Geometry check sheet. Reference: the model listing, model coordinates, mm. A direction names the side the tool comes from. Coordinates: 2 decimals unless noted, no trailing zeros. Loops run counter-clockwise (first coordinate to the right, second up) from the corner with the lowest first, then second, coordinate; pieces in that order, holes last. Notation, with made-up numbers: (14, 30) - (55, 30) arc R17 cw to (55, 47) - close; hole circle Ø3 at (58, 22). An arc over 180 degrees is marked (long way). Write each question's results on one line, items separated by ' | '. Start each with the question number.
(1) Sectioned sample at D-D (y = 32.5). Enter the section's corners in (x, z), plus the area to 3 significant figures.
(2) Material ranges on probe 1 along Y at (x, z) = (50, 9); probe 2 along X at (y, z) = (68, 27.5); probe 3 along Y at (x, z) = (24.5, 2.5), recorded low to high.
(3) Mould release check, pull along Y, two halves, no side actions. Record for faces 1 (the face through (55, 78, 16)), 2 (the face through (53, 45, 17)), 3 (the face through (23, 41, -4)), 4 (the face through (54, 11, 16)): pulls with the +Y half, pulls with the -Y half, needs draft (parallel to the pull), parting line crosses it, or undercut.
(4) Go/stop test with flat-tipped pins: pin 1 Ø2 at (x, y) = (38.5, 66.5) entering from +Z; pin 2 Ø7.5 at (x, z) = (-5, 10.5) entering from -Y; pin 3 Ø5.5 at (x, z) = (48.5, 21) entering from -Y. Record where each tip stops, or that it passes through.
(5) Sectioned sample at C-C (x = 32). Enter the section's corners in (y, z), plus the area to 3 significant figures.
(6) Sectioned sample at B-B (z = 14.5). State how many separate pieces and enclosed holes the cut face has, plus the area to 3 significant figures.
(7) Sectioned sample at A-A (y = 74). Enter the section's corners in (x, z).
(8) Access from +Z, -Z, +X, -X, +Y, -Y to the whole of each face (thin tool, end or side, straight path). Record for faces 5 (the face through (50, 76, 17)), 6 (the face through (23, 0, 16)), 7 (the face through (46.2, 7, 16)).
from build123d import *

# Parameters (mm, degrees)
F0_R     = 2
F1_DEPTH = 35
F2_DEPTH = 4


with BuildPart() as f1:
    # F0 (on Top) → F1 (new body)
    with BuildSketch(Plane.XY):
        with BuildLine():
            ThreePointArc((-0.098751, 4.899238), (1.400506, 1.429019), (4.900234, 0))
            Line((4.900234, 0), (41.2, 0))
            ThreePointArc((41.2, 0), (44.735534, 1.464466), (46.2, 5))
            Line((46.2, 5), (46.2, 10))
            Line((46.2, 10), (51, 10))
            ThreePointArc((51, 10), (54.535534, 11.464466), (56, 15))
            Line((56, 15), (56, 30))
            Line((56, 30), (56, 75))
            ThreePointArc((56, 75), (54.535534, 78.535534), (51, 80))
            Line((51, 80), (-5, 80))
            ThreePointArc((-5, 80), (-8.535534, 78.535534), (-10, 75))
            Line((-10, 75), (-10, 30))
            Line((-10, 30), (-10, 15))
            ThreePointArc((-10, 15), (-8.535534, 11.464466), (-5, 10))
            Line((-5, 10), (-0.201564, 10))
            Line((-0.201564, 10), (-0.098751, 4.899238))
        make_face()
        with Locations((-4, 16)):
            Circle(F0_R, mode=Mode.SUBTRACT)
        with Locations((50, 16)):
            Circle(F0_R, mode=Mode.SUBTRACT)
        with Locations((-4, 74)):
            Circle(F0_R, mode=Mode.SUBTRACT)
        Polygon((-7, 30), (-7, 70), (0, 70), (0, 77), (23, 77), (46, 77), (46, 70), (53, 70), (53, 30), (53, 20), (46.201564, 20), (43.202173, 10.060457), (43.09936, 4.959695), (41.099766, 3), (23.1, 3), (22.9, 3), (4.900234, 3), (2.90064, 4.959695), (2.797827, 10.060457), (-0.201564, 20), (-7, 20), align=None, mode=Mode.SUBTRACT)
        with Locations((50, 74)):
            Circle(F0_R, mode=Mode.SUBTRACT)
    extrude(amount=F1_DEPTH)

    # F0 (on Top) → F2 (join)
    with BuildSketch(Plane.XY):
        with BuildLine():
            ThreePointArc((-0.098751, 4.899238), (1.400506, 1.429019), (4.900234, 0))
            Line((4.900234, 0), (41.2, 0))
            ThreePointArc((41.2, 0), (44.735534, 1.464466), (46.2, 5))
            Line((46.2, 5), (46.2, 10))
            Line((46.2, 10), (51, 10))
            ThreePointArc((51, 10), (54.535534, 11.464466), (56, 15))
            Line((56, 15), (56, 30))
            Line((56, 30), (56, 75))
            ThreePointArc((56, 75), (54.535534, 78.535534), (51, 80))
            Line((51, 80), (-5, 80))
            ThreePointArc((-5, 80), (-8.535534, 78.535534), (-10, 75))
            Line((-10, 75), (-10, 30))
            Line((-10, 30), (-10, 15))
            ThreePointArc((-10, 15), (-8.535534, 11.464466), (-5, 10))
            Line((-5, 10), (-0.201564, 10))
            Line((-0.201564, 10), (-0.098751, 4.899238))
        make_face()
        with Locations((-4, 16)):
            Circle(F0_R, mode=Mode.SUBTRACT)
        with Locations((50, 16)):
            Circle(F0_R, mode=Mode.SUBTRACT)
        with Locations((-4, 74)):
            Circle(F0_R, mode=Mode.SUBTRACT)
        Polygon((-7, 30), (-7, 70), (0, 70), (0, 77), (23, 77), (46, 77), (46, 70), (53, 70), (53, 30), (53, 20), (46.201564, 20), (43.202173, 10.060457), (43.09936, 4.959695), (41.099766, 3), (23.1, 3), (22.9, 3), (4.900234, 3), (2.90064, 4.959695), (2.797827, 10.060457), (-0.201564, 20), (-7, 20), align=None, mode=Mode.SUBTRACT)
        with Locations((50, 74)):
            Circle(F0_R, mode=Mode.SUBTRACT)
        Polygon((0, 70), (-7, 70), (-7, 30), (-7, 20), (-0.201564, 20), (2.797827, 10.060457), (2.90064, 4.959695), (4.900234, 3), (22.9, 3), (23.1, 3), (41.099766, 3), (43.09936, 4.959695), (43.202173, 10.060457), (46.201564, 20), (53, 20), (53, 30), (53, 70), (46, 70), (46, 77), (23, 77), (0, 77), align=None)
        with Locations((50, 74)):
            Circle(F0_R)
        with Locations((-4, 74)):
            Circle(F0_R)
        with Locations((-4, 16)):
            Circle(F0_R)
        with Locations((50, 16)):
            Circle(F0_R)
    extrude(amount=-F2_DEPTH)


solid = f1.part
Outcome:
1) outline: (-10, -4) - (56, -4) - (56, 35) - (53, 35) - (53, 0) - (-7, 0) - (-7, 35) - (-10, 35) - close | area: 474 mm2
2) probe 1: y = 10 to 14, 18 to 20, 70 to 72, 76 to 80 | probe 2: x = -10 to -7, 53 to 56 | probe 3: y = 0 to 3, 77 to 80
3) face 1: pulls with the +Y half | face 2: undercut | face 3: needs draft | face 4: pulls with the -Y half
4) pin 1: stops at z = 0 | pin 2: stops at y = 10 | pin 3: stops at y = 2.93
5) outline: (0, -4) - (80, -4) - (80, 35) - (77, 35) - (77, 0) - (3, 0) - (3, 35) - (0, 35) - close | area: 530 mm2
6) separate pieces: 1 | enclosed holes: 5 | area: 967 mm2
7) outline: (-10, -4) - (56, -4) - (56, 35) - (52, 35) - (52, 0) - (48, 0) - (48, 35) - (46, 35) - (46, 0) - (0, 0) - (0, 35) - (-2, 35) - (-2, 0) - (-6, 0) - (-6, 35) - (-10, 35) - close
8) face 5: +Z | face 6: +Z, -Z, +X, -X, -Y | face 7: +Z, -Z, +X, -Y
